from build123d import *

# Parameters (mm, degrees)
SKETCH1_W           = 40
SKETCH1_H           = 100
BOSS_EXTRUDE1_DEPTH = 5
SKETCH2_W           = 20
SKETCH2_H           = 5
BOSS_EXTRUDE2_DEPTH = 5
SKETCH3_R           = 6
BOSS_EXTRUDE3_DEPTH = 5
SKETCH4_R           = 2.5
CUT_EXTRUDE1_DEPTH  = 5


with BuildPart() as part:
    # Sketch1 → Boss-Extrude1 (new body)
    with BuildSketch(Plane.XY):
        Rectangle(SKETCH1_W, SKETCH1_H)
    extrude(amount=BOSS_EXTRUDE1_DEPTH)

    # Sketch2 → Boss-Extrude2 (add)
    with BuildSketch(Plane(origin=(0, 50, 0), x_dir=(1, 0, 0), z_dir=(0, 1, 0))):
        with Locations((0, -2.5)):
            Rectangle(SKETCH2_W, SKETCH2_H)
    boss_extrude2 = extrude(amount=BOSS_EXTRUDE2_DEPTH)

    # Mirror1: Boss-Extrude2 across plane
    add(boss_extrude2.mirror(Plane.ZX))

    # Sketch3 → Boss-Extrude3 (add)
    with BuildSketch(Plane.XY.offset(5)):
        with Locations((0, 52.5)):
            Circle(SKETCH3_R)
    boss_extrude3 = extrude(amount=-BOSS_EXTRUDE3_DEPTH)

    # Sketch4 → Cut-Extrude1 (cut)
    with BuildSketch(Plane.XY.offset(5)):
        with Locations((0, 52.5)):
            Circle(SKETCH4_R)
    cut_extrude1 = extrude(amount=-CUT_EXTRUDE1_DEPTH, mode=Mode.SUBTRACT)

    # Mirror2: Boss-Extrude3, Cut-Extrude1 across plane
    add(boss_extrude3.mirror(Plane.ZX))
    add(cut_extrude1.mirror(Plane.ZX), mode=Mode.SUBTRACT)


solid = part.part
Read the model definition and answer for the solid it produces. Units are mm, in the model's axes. A direction names the side the tool comes from. Round coordinates to 2 decimals unless told otherwise and drop trailing zeros. Loops run counter-clockwise (first coordinate to the right, second up) from the corner with the lowest first, then second, coordinate; pieces in that order, holes last.
Q1. Determine the mould class of faces 1 (the face through (10, -52, 3)), 2 (the face through (8, -55, 2)), 3 (the face through (-0.54, -50.06, 2.54)) for opening direction X: released by +X, released by -X, zero draft, split by the parting line, or undercut.
Q2. Section A-A on y = 52.5 is taken. Write down the section's boundary in (x, z), and give its area (3 significant figures).
Q3. Each of these flat-tipped pins is pushed along its axis until it touches: pin 1 (2.5 mm diameter, centred on x = 8, z = 2, fed in from +Y); pin 2 (2.5 mm diameter, centred on y = 53.5, z = 2.5, fed in from +X); pin 3 (2.5 mm diameter, centred on y = 52.5, z = 2, fed in from -X). Where does it stop, or does it pass through?
Q4. Section D-D on x = -7 is taken. Write down the section's boundary in (y, z), and give its area (3 significant figures).
Q5. Section B-B on x = 0 is taken. Write down the section's boundary in (y, z), and give its area (3 significant figures).
Q6. Consider probe 1 along Y at (x, z) = (0, 2.75); probe 2 along X at (y, z) = (-52.5, 1.7); probe 3 along Y at (x, z) = (-15.5, 2.7). Determine where each line is inside the solid, lowest interval first.
Q7. Section C-C on z = 1 is taken. Write down the section's boundary in (x, y), and give its area (3 significant figures).
Q8. Which of the six approach directions +Z, -Z, +X, -X, +Y, -Y give full straight-line access (tool end or side, diameter ignored) to faces 4 (the face through (-0.54, 50.06, 2.54)), 5 (the face through (8, 55, 2)), 6 (the face through (-10, -52, 3)), 7 (the face through (-10, 52, 3))?
Output:
1. face 1: released by +X
1. face 2: zero draft
1. face 3: undercut
2. outline: (-10, 0) - (-2.5, 0) - (-2.5, 5) - (-10, 5) - close; (2.5, 0) - (10, 0) - (10, 5) - (2.5, 5) - close
2. area: 75.0 mm2
3. pin 1: stops at y = 55
3. pin 2: stops at x = 10
3. pin 3: stops at x = -10
4. outline: (-55, 0) - (55, 0) - (55, 5) - (-55, 5) - close
4. area: 550 mm2
5. outline: (-58.5, 0) - (-55, 0) - (-55, 5) - (-58.5, 5) - close; (-50, 0) - (50, 0) - (50, 5) - (-50, 5) - close; (55, 0) - (58.5, 0) - (58.5, 5) - (55, 5) - close
5. area: 535 mm2
6. probe 1: y = -58.5 to -55, -50 to 50, 55 to 58.5
6. probe 2: x = -10 to -2.5, 2.5 to 10
6. probe 3: y = -50 to 50
7. outline: (-20, -50) - (-10, -50) - (-10, -55) - (-5.45, -55) arc R6 ccw to (5.45, -55) - (10, -55) - (10, -50) - (20, -50) - (20, 50) - (10, 50) - (10, 55) - (5.45, 55) arc R6 ccw to (-5.45, 55) - (-10, 55) - (-10, 50) - (-20, 50) - close; hole circle Ø5 at (0, -52.5); hole circle Ø5 at (0, 52.5)
7. area: 4,220 mm2
8. face 4: +Z, -Z
8. face 5: +Z, -Z, +X, +Y
8. face 6: +Z, -Z, -X, -Y
8. face 7: +Z, -Z, -X, +Y
